```python
from build123d import *

# Parameters (mm, degrees)
F1_DEPTH = 9
F2_R     = 1.75
F3_DEPTH = 25
F4_R     = 4
F5_ANGLE = 90


with BuildPart() as f1:
    # F0 (on Top) → F1 (new body)
    with BuildSketch(Plane.XY):
        Polygon((-11, 1), (-11, 0), (11, 0), (11, 1), (5.5, 1), (5.5, 10), (2.5, 10), (2.5, 1), (-2.5, 1), (-2.5, 10), (-5.5, 10), (-5.5, 1), align=None)
    extrude(amount=F1_DEPTH)

    # F2 (on face) → F3 (cut)
    with BuildSketch(Plane.YZ.offset(5.5)):
        with Locations((5.5, 4.5)):
            Circle(F2_R)
    extrude(amount=-F3_DEPTH, mode=Mode.SUBTRACT)

    # F4
    f4_edges = [f1.edges().sort_by_distance(p)[0] for p in [
        (-4, 10, 9),
        (4, 10, 9),
        (4, 10, 0),
        (-4, 10, 0),
    ]]
    fillet(f4_edges, radius=F4_R)


with BuildPart() as f1_1:
    # F5: moved
    add(f1.part.rotate(Axis((0, 0, 0), (1, 0, 0)), F5_ANGLE))


solid = f1_1.part
```
Source: CAD feature listing. Evaluate the final solid. Frame: model axes, mm. A direction names the side the tool comes from. Round coordinates to 2 decimals unless told otherwise and drop trailing zeros. Loops run counter-clockwise (first coordinate to the right, second up) from the corner with the lowest first, then second, coordinate; pieces in that order, holes last.
1. Section query C-C on z = 5.5. Output: boundary loops of the cut face in (x, y), and give its area (3 significant figures).
2. Section query A-A on z = 2. Output: boundary loops of the cut face in (x, y).
3. Contact query for flat-ended pins moving along their axis: pin 1 (4.5 mm diameter, centred on y = -4.5, z = 5.5, fed in from +X); pin 2 (3 mm diameter, centred on x = 9, y = -3.5, fed in from +Z); pin 3 (4.5 mm diameter, centred on y = -3, z = 4.5, fed in from -X). Output: stop coordinate, or through.
4. Ray query, L1, parallel to X at y = -6, z = 2.5; L2, parallel to Y at x = -4.5, z = 5.5; L3, parallel to Z at x = 10, y = -2.75. Return the intervals inside material, ascending.
5. Section query D-D on y = -3. Output: boundary loops of the cut face in (x, z).
6. Access query for faces 1 (the flat face through (5.5, -4, 3)), 2 (the flat face through (-8, -4, 1)), 3 (the flat face through (-2.5, -4, 3)). Directions: +Z, -Z, +X, -X, +Y, -Y. A direction counts if a zero-diameter tool reaches every point of the face in a straight line with its end or side. Return the directions, or none.
7. Section query B-B on y = -4.5. Output: boundary loops of the cut face in (x, z).
8. Mould query, pull axis Y, two halves, no side actions, for faces 4 (the cylindrical face through (4.02, -2.79, 5.12)), 5 (the flat face through (-11, -4.4, 0.5)), 6 (the flat face through (-3, 0, 2)). Classes: released by +Y, released by -Y, zero draft, split by the parting line, or undercut.
Answers below:
1. outline: (-5.5, -9) - (-2.5, -9) - (-2.5, -6.25) - (-5.5, -6.25) - close; (-5.5, -2.75) - (-2.5, -2.75) - (-2.5, 0) - (-5.5, 0) - close; (2.5, -9) - (5.5, -9) - (5.5, -6.25) - (2.5, -6.25) - close; (2.5, -2.75) - (5.5, -2.75) - (5.5, 0) - (2.5, 0) - close
1. area: 33.0 mm2
2. outline: (-5.5, -9) - (-2.5, -9) - (-2.5, 0) - (-5.5, 0) - close; (2.5, -9) - (5.5, -9) - (5.5, 0) - (2.5, 0) - close
3. pin 1: stops at x = 5.5
3. pin 2: stops at z = 1
3. pin 3: stops at x = -5.5
4. L1: x = -5.5 to -2.5, 2.5 to 5.5
4. L2: y = -9 to -6.25, -2.75 to 0
4. L3: z = 0 to 1
5. outline: (-11, 0) - (11, 0) - (11, 1) - (5.5, 1) - (5.5, 4.6) - (2.5, 4.6) - (2.5, 1) - (-2.5, 1) - (-2.5, 4.6) - (-5.5, 4.6) - (-5.5, 1) - (-11, 1) - close; (-5.5, 6.4) - (-2.5, 6.4) - (-2.5, 9.87) - (-5.5, 9.87) - close; (2.5, 6.4) - (5.5, 6.4) - (5.5, 9.87) - (2.5, 9.87) - close
6. face 1: +Z, +X, +Y, -Y
6. face 2: +Z, -X, +Y, -Y
6. face 3: +Z, +Y, -Y
7. outline: (-11, 0) - (11, 0) - (11, 1) - (5.5, 1) - (5.5, 3.75) - (2.5, 3.75) - (2.5, 1) - (-2.5, 1) - (-2.5, 3.75) - (-5.5, 3.75) - (-5.5, 1) - (-11, 1) - close; (-5.5, 7.25) - (-2.5, 7.25) - (-2.5, 10) - (-5.5, 10) - close; (2.5, 7.25) - (5.5, 7.25) - (5.5, 10) - (2.5, 10) - close
8. face 4: undercut
8. face 5: zero draft
8. face 6: released by +Y
